from build123d import *
from build123d import SkipClean  # not in build123d's __all__

# Parameters (mm, degrees)
F2_R      = 15
F3_DEPTH  = 100
F4_R      = 10
F5_DEPTH  = 25
F6_R      = 15
F7_DEPTH  = 85
F8_R      = 10
F9_DEPTH  = 25
F10_R     = 15
F11_DEPTH = 85
F12_R     = 10
F13_DEPTH = 25


with BuildPart() as f3:
    # F2 (on Front) → F3 (new body)
    with BuildSketch(Plane.XZ):
        Circle(F2_R)
    extrude(amount=F3_DEPTH)

    # F4 (on face) → F5 (cut)
    with BuildSketch(Plane.XZ.offset(100)):
        Circle(F4_R)
    extrude(amount=-F5_DEPTH, mode=Mode.SUBTRACT)

    # F6 (on Top) → F7 (join)
    with BuildSketch(Plane.XY):
        with Locations((0, -15)):
            Circle(F6_R)
    with SkipClean():  # cleaning this boolean's faces spoils the solid; the shape is the same uncleaned
        extrude(amount=F7_DEPTH)

    # F8 (on face) → F9 (cut)
    with BuildSketch(Plane.XY.offset(85)):
        with Locations((0, -15)):
            Circle(F8_R)
    with SkipClean():  # cleaning this boolean's faces spoils the solid; the shape is the same uncleaned
        extrude(amount=-F9_DEPTH, mode=Mode.SUBTRACT)

    # F10 (on Right) → F11 (join)
    with BuildSketch(Plane.YZ):
        with Locations((-15, 0)):
            Circle(F10_R)
    extrude(amount=F11_DEPTH)

    # F12 (on face) → F13 (cut)
    with BuildSketch(Plane.YZ.offset(85)):
        with Locations((-15, 0)):
            Circle(F12_R)
    extrude(amount=-F13_DEPTH, mode=Mode.SUBTRACT)


solid = f3.part
The listing builds one solid part. Answer for the finished solid, in the listing's coordinates (mm). A direction names the side the tool comes from. Coordinates: 2 decimals unless noted, no trailing zeros. Order: outer loops, then holes, each group sorted by start corner. A loop starts at its lowest first (then second) coordinate and runs counter-clockwise, first axis right, second up. Notation, with made-up numbers: (-5.75, -38.75) -> (49.25, -38.75) arc R33 cw to (49.25, -1.75) -> close; hole circle Ø11 at (-28.5, -6). An arc over 180 degrees is marked (long way). Answer in a Markdown table with one row per item. Add a question column.
Item 1: Find the intervals of material crossed by L1, parallel to Z at x = 75, y = -15; L2, parallel to Y at x = 6.5, z = 63.5; L3, parallel to Y at x = 29.5, z = 0.5, in increasing order. Write a range as from..to.
Item 2: Find section C-C (x = -3). Write down the section's boundary in (y, z), then the cut area to 3 significant figures.
Item 3: Which of the six approach directions +Z, -Z, +X, -X, +Y, -Y give full straight-line access (tool end or side, diameter ignored) to faces 1 (the face through (10.645, -1.373, 10.568)), 2 (the face through (-2.17, -87.68, -9.76)), 3 (the face through (-14.985, -14.34, 51.349)), 4 (the face through (72.68, -5.46, 3))?
Item 4: Find section A-A (y = -15). Write down the section's boundary in (x, z).
Item 5: Find section D-D (x = 61.5). Write down the section's boundary in (y, z), then the cut area to 3 significant figures.
Item 6: Each of these flat-tipped pins is pushed along its axis until it touches: P1, Ø12, axis at x = 23.5, y = -73.5, coming from the -Z side; P2, Ø8, axis at x = 16.5, y = -87.5, coming from the +Z side; P3, Ø1, axis at y = -19.5, z = 61.5, coming from the +X side; P4, Ø4, axis at x = 6.5, y = -33, coming from the -Z side. Where does it stop, or does it pass through?
Item 7: Find section B-B (z = 66.5). Write down the section's boundary in (x, y).
Item 8: Determine the mould class of faces 5 (the face through (51.349, -18.252, -14.643)), 6 (the face through (0, -15, 60)), 7 (the face through (0, 0, 0)) for opening direction Y: +Y half, -Y half, draft (parallel to the pull), parting line (faces both ways), or undercut.
Result set:
| question | item | result |
|---|---|---|
| 1 | L1 | z = -15..-10, 10..15 |
| 1 | L2 | y = -28.52..-22.6, -7.4..-1.48 |
| 1 | L3 | y = -29.99..-0.01 |
| 2 | outline | (-100, -14.7) -> (0, -14.7) -> (0, 14.7) -> (-0.3, 14.7) -> (-0.3, 85) -> (-5.46, 85) -> (-5.46, 60) -> (-24.54, 60) -> (-24.54, 85) -> (-29.7, 85) -> (-29.7, 14.7) -> (-100, 14.7) -> (-100, 9.54) -> (-75, 9.54) -> (-75, -9.54) -> (-100, -9.54) -> close |
| 2 | area | 4,050 mm² |
| 3 | face 1 | +Z, +X, +Y |
| 3 | face 2 | -Y |
| 3 | face 3 | +Z |
| 3 | face 4 | +X |
| 4 | outline | (-15, 0) arc R15 ccw to (0, -15) -> (85, -15) -> (85, -10) -> (60, -10) -> (60, 10) -> (85, 10) -> (85, 15) -> (15, 15) -> (15, 85) -> (10, 85) -> (10, 60) -> (-10, 60) -> (-10, 85) -> (-15, 85) -> close |
| 5 | outline | circle Ø30 at (-15, 0); hole circle Ø20 at (-15, 0) |
| 5 | area | 393 mm² |
| 6 | P1 | passes through |
| 6 | P2 | stops at z = 8.29 |
| 6 | P3 | stops at x = 14.46 |
| 6 | P4 | stops at z = -14.31 |
| 7 | outline | circle Ø30 at (0, -15); hole circle Ø20 at (0, -15) |
| 8 | face 5 | parting line |
| 8 | face 6 | undercut |
| 8 | face 7 | +Y half |
